CAD build for the part. Positions are in the model's coordinates, mm. A direction names the side the tool comes from. Coordinates: 2 decimals unless noted, no trailing zeros. Order: outer loops, then holes, each group sorted by start corner. A loop starts at its lowest first (then second) coordinate and runs counter-clockwise, first axis right, second up.
from build123d import *

# Parameters (mm, degrees)
SKETCH1_W           = 15
SKETCH1_H           = 1
SKETCH1_W_2         = 1
SKETCH1_H_2         = 14
BOSS_EXTRUDE1_DEPTH = 8
SKETCH2_R           = 1.5
CUT_EXTRUDE1_DEPTH  = 16
SKETCH3_R           = 1.5
CUT_EXTRUDE2_DEPTH  = 16


with BuildPart() as part:
    # Sketch1 → Boss-Extrude1 (new body)
    with BuildSketch(Plane.XY):
        Rectangle(SKETCH1_W, SKETCH1_H)
        with Locations((7, -7.5)):
            Rectangle(SKETCH1_W_2, SKETCH1_H_2)
    extrude(amount=BOSS_EXTRUDE1_DEPTH)

    # Sketch2 → Cut-Extrude1 (cut, through all)
    with BuildSketch(Plane(origin=(0, 0.5, 0), x_dir=(1, 0, 0), z_dir=(0, 1, 0))):
        with Locations((-3.5, -4)):
            Circle(SKETCH2_R)
        with Locations((3.5, -4)):
            Circle(SKETCH2_R)
    extrude(amount=-CUT_EXTRUDE1_DEPTH, mode=Mode.SUBTRACT)

    # Sketch3 → Cut-Extrude2 (cut, through all)
    with BuildSketch(Plane(origin=(7.5, 0, 0), x_dir=(0, 0, -1), z_dir=(1, 0, 0))):
        with Locations((-4, -3.5)):
            Circle(SKETCH3_R)
        with Locations((-4, -10.5)):
            Circle(SKETCH3_R)
    extrude(amount=-CUT_EXTRUDE2_DEPTH, mode=Mode.SUBTRACT)


solid = part.part
1) Drill centre lines: probe 1 along X at (y, z) = (0.3, 4); probe 2 along Y at (x, z) = (7.3, 4); probe 3 along Z at (x, y) = (-3.5, -0.3). Where is each one in solid material? Low to high.
2) Two-plate mould, pull along Z, no slides. Class faces 1 (the flat face through (3, 0, 0)), 2 (the flat face through (7, -14.5, 4)), 3 (the cylindrical face through (-2, 0, 4)): released by +Z, released by -Z, zero draft, split by the parting line, or undercut.
3) Pin check, flat tips, straight feed: P1, Ø3, axis at y = -4, z = 2.5, coming from the -X side; P2, Ø2.5, axis at x = -3.5, z = 4, coming from the -Y side. Stop position of each tip, or through.
4) Slice it at B-B (z = 4). List the corners of the cut face in (x, y), plus the area to 3 significant figures.
5) Slice it at C-C (y = -10.5). List the corners of the cut face in (x, z).
6) Which spindle directions (+Z, -Z, +X, -X, +Y, -Y) get a long thin tool onto all of the face, cutting with end or side? Do faces 4 (the cylindrical face through (7.01, -11.83, 3.31)), 5 (the flat face through (-1, -0.5, 4)). Say none if no direction does.
7) Slice it at D-D (z = 1.75). List the corners of the cut face in (x, y).
8) Slice it at A-A (x = 3.5). List the corners of the cut face in (y, z), plus the area to 3 significant figures.
Worked out:
1. probe 1: x = -7.5 to -5, -2 to 2, 5 to 7.5
1. probe 2: y = -14.5 to -12, -9 to -5, -2 to 0.5
1. probe 3: z = 0 to 2.5, 5.5 to 8
2. face 1: released by -Z
2. face 2: zero draft
2. face 3: undercut
3. P1: stops at x = 6.5
3. P2: passes through
4. outline: (-7.5, -0.5) - (-5, -0.5) - (-5, 0.5) - (-7.5, 0.5) - close; (-2, -0.5) - (2, -0.5) - (2, 0.5) - (-2, 0.5) - close; (5, -0.5) - (6.5, -0.5) - (6.5, -2) - (7.5, -2) - (7.5, 0.5) - (5, 0.5) - close; (6.5, -14.5) - (7.5, -14.5) - (7.5, -12) - (6.5, -12) - close; (6.5, -9) - (7.5, -9) - (7.5, -5) - (6.5, -5) - close
4. area: 17.0 mm2
5. outline: (6.5, 0) - (7.5, 0) - (7.5, 2.5) - (6.5, 2.5) - close; (6.5, 5.5) - (7.5, 5.5) - (7.5, 8) - (6.5, 8) - close
6. face 4: +X, -X
6. face 5: +Z, -Z, -X, -Y
7. outline: (-7.5, -0.5) - (6.5, -0.5) - (6.5, -14.5) - (7.5, -14.5) - (7.5, 0.5) - (-7.5, 0.5) - close
8. outline: (-0.5, 0) - (0.5, 0) - (0.5, 2.5) - (-0.5, 2.5) - close; (-0.5, 5.5) - (0.5, 5.5) - (0.5, 8) - (-0.5, 8) - close
8. area: 5.00 mm2
